Can you work these out from the drawing? Everything is in mm from the part's minimum corner. A direction names the side the tool comes from. Round coordinates to 2 decimals unless told otherwise and drop trailing zeros. Write each loop counter-clockwise with the first axis right and the second up, starting at its lowest first coordinate (ties: lowest second). Pieces come first, ordered by that corner, then holes. Notation, with made-up numbers: (33.5, 70) - (80.5, 70) arc R24 cw to (80.5, 103) - close; hole circle Ø10 at (80, -35). An arc over 180 degrees is marked (long way). One line per item, written item: value. Start each with the question number.
Item 1: For P1, Ø1, axis at y = 9, z = 10.5, coming from the +X side; P2, Ø5, axis at x = 7, y = 7, coming from the +Z side; P3, Ø3.5, axis at x = 14.5, y = 9, coming from the +Z side, each with a flat end and sliding along its axis, tell me the tip position at first contact or that it passes through.
Item 2: Imagine slicing it at D-D, the plane x = 5.25. Please give me the cut outline in (y, z), then the cut area to 3 significant figures.
Item 3: Imagine slicing it at A-A, the plane z = 4.75. Please give me the cut outline in (x, y), then the cut area to 3 significant figures.
Item 4: For the marked faces 1, 2 and 3, which set-ups out of +Z, -Z, +X, -X, +Y, -Y let a thin tool reach every point of the face, with its end or its side?
Item 5: Imagine slicing it at C-C, the plane y = 5.5. Please give me the cut outline in (x, z), then the cut area to 3 significant figures.
Item 6: If I drill on line 1 (X direction, y = 5, z = 8.75); line 2 (Z direction, x = 21, y = 16.5); line 3 (Y direction, x = 18.25, z = 9.75) (1 decimal), over which ranges is the centre line in solid material (lowest first)?
Item 7: Imagine slicing it at B-B, the plane z = 9. Please give me the cut outline in (x, y).
Item 8: Thinking about a two-plate mould opening in X: for the marked faces 4, 5, 6 and 7, which applies, released by +X, released by -X, zero draft, split by the parting line, or undercut?
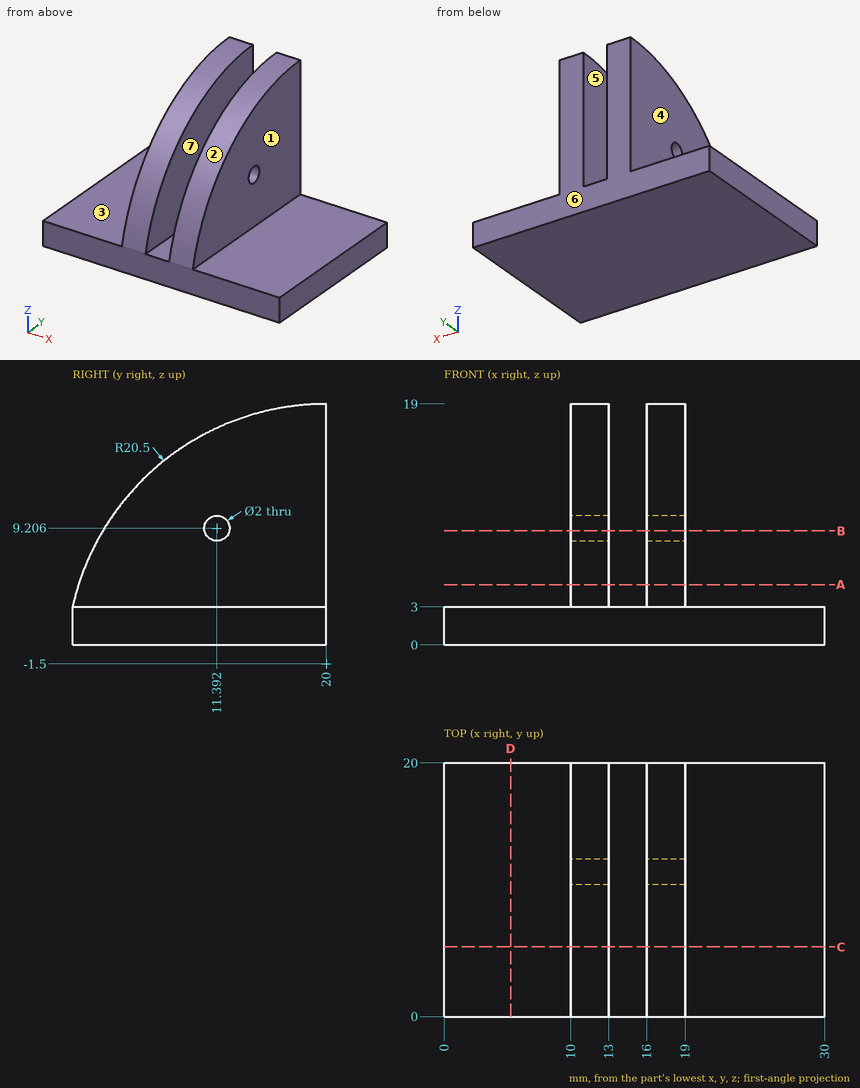
Values follow:
1. P1: stops at x = 19
1. P2: stops at z = 3
1. P3: stops at z = 16.34
2. outline: (0, 0) - (20, 0) - (20, 3) - (0, 3) - close
2. area: 60.0 mm^2
3. outline: (10, 0.48) - (13, 0.48) - (13, 20) - (10, 20) - close; (16, 0.48) - (19, 0.48) - (19, 20) - (16, 20) - close
3. area: 117 mm^2
4. face 1: +Z, +X, +Y, -Y
4. face 2: +Z, +X, -X, -Y
4. face 3: +Z, -X, +Y, -Y
5. outline: (0, 0) - (30, 0) - (30, 3) - (19, 3) - (19, 12.99) - (16, 12.99) - (16, 3) - (13, 3) - (13, 12.99) - (10, 12.99) - (10, 3) - (0, 3) - close
5. area: 150 mm^2
6. line 1: x = 10 to 13, 16 to 19
6. line 2: z = 0 to 3
6. line 3: y = 2.9 to 10.6, 12.2 to 20
7. outline: (10, 2.39) - (13, 2.39) - (13, 10.41) - (10, 10.41) - close; (10, 12.37) - (13, 12.37) - (13, 20) - (10, 20) - close; (16, 2.39) - (19, 2.39) - (19, 10.41) - (16, 10.41) - close; (16, 12.37) - (19, 12.37) - (19, 20) - (16, 20) - close
8. face 4: released by -X
8. face 5: undercut
8. face 6: zero draft
8. face 7: undercut
